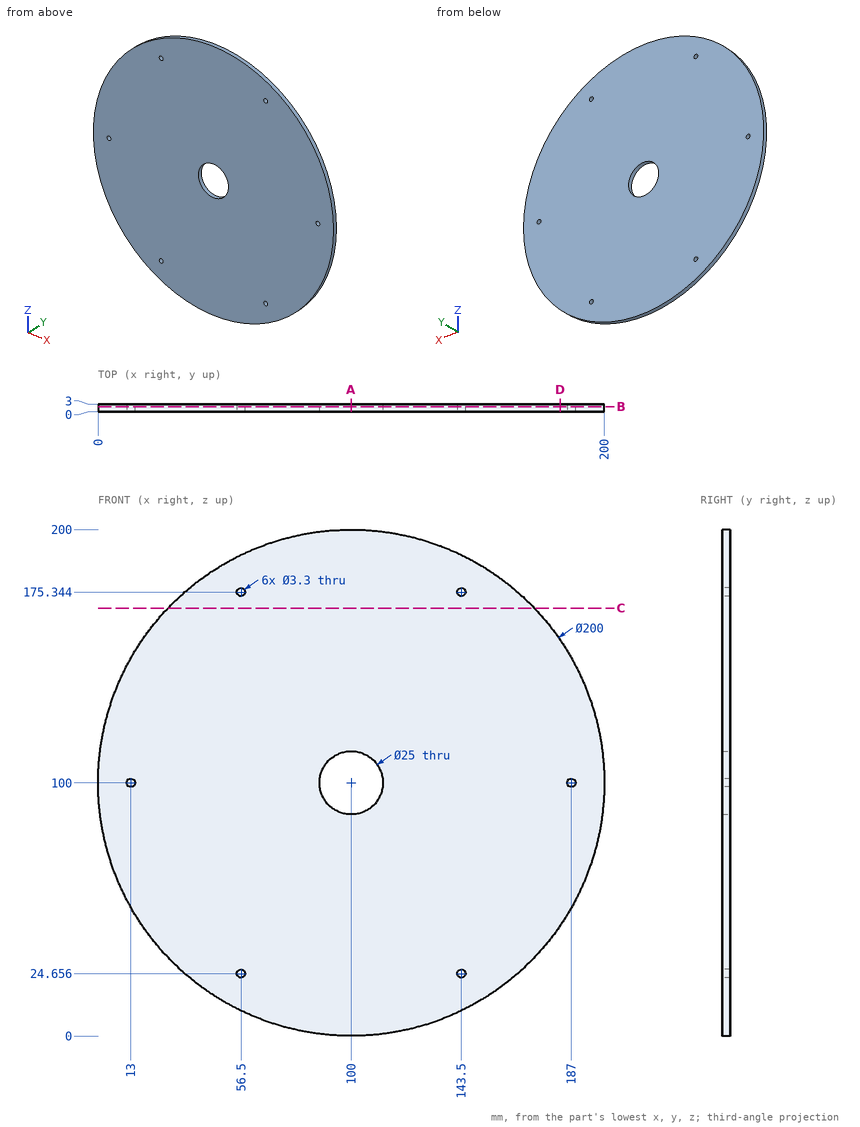
Could you check a few things on this drawing? It's one solid part, dimensions in mm from its lowest x, y, z. Coordinates: 2 decimals unless noted, no trailing zeros. Order: outer loops, then holes, each group sorted by start corner. A loop starts at its lowest first (then second) coordinate and runs counter-clockwise, first axis right, second up.
1) I need wall thicknesses on line 1 (Z direction, x = 100, y = 2.25); line 2 (Z direction, x = 143.5, y = 1.95) (1 decimal); line 3 (Z direction, x = 101.5, y = 1.6). Which ranges of each line are inside material? Lowest first, please.
2) Imagine slicing it at A-A on x = 100. List the corners of the cut face in (y, z) for me, and give its area (3 significant figures).
3) Imagine slicing it at C-C on z = 169. List the corners of the cut face in (x, y) for me, and give its area (3 significant figures).
4) Will these pins go through, and if not, where does the flat tip stop? pin 1 (1 mm diameter, centred on x = 119, y = 1.5, fed in from +Z); pin 2 (1 mm diameter, centred on y = 1.5, z = 21.5, fed in from +X).
5) Imagine slicing it at B-B on y = 2. List the corners of the cut face in (x, z) for me.
6) Imagine slicing it at D-D on x = 182.5. List the corners of the cut face in (y, z) for me.
Response values:
1. line 1: z = 0 to 87.5, 112.5 to 200
1. line 2: z = 10 to 23, 26.3 to 173.7, 177 to 190
1. line 3: z = 0.01 to 87.59, 112.41 to 199.99
2. outline: (0, 0) - (3, 0) - (3, 87.5) - (0, 87.5) - close; (0, 112.5) - (3, 112.5) - (3, 200) - (0, 200) - close
2. area: 525 mm2
3. outline: (27.62, 0) - (172.38, 0) - (172.38, 3) - (27.62, 3) - close
3. area: 434 mm2
4. pin 1: stops at z = 198.27
4. pin 2: stops at x = 162.58
5. outline: circle Ø200 at (100, 100); hole circle Ø3.3 at (13, 100); hole circle Ø3.3 at (56.5, 24.66); hole circle Ø3.3 at (56.5, 175.34); hole circle Ø25 at (100, 100); hole circle Ø3.3 at (143.5, 24.66); hole circle Ø3.3 at (143.5, 175.34); hole circle Ø3.3 at (187, 100)
6. outline: (0, 43.49) - (3, 43.49) - (3, 156.51) - (0, 156.51) - close
